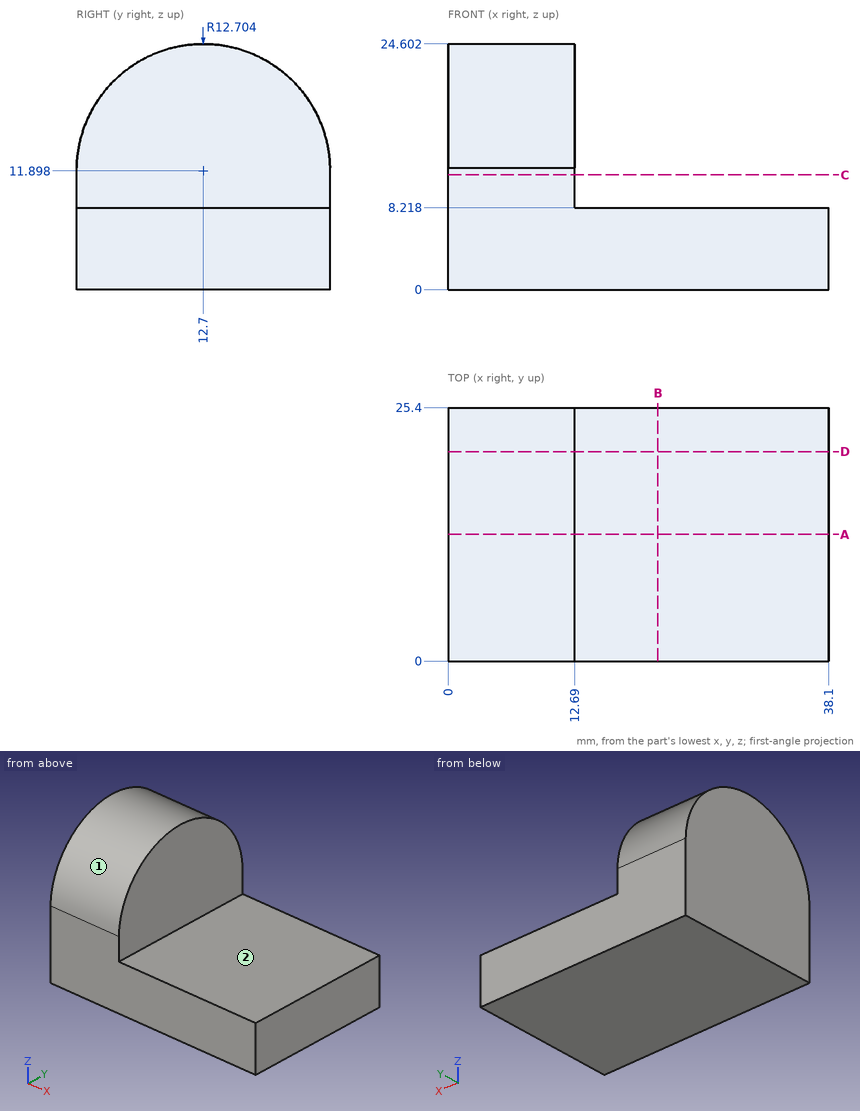
Answer from the drawing. Dimensions are ordinates in mm from the lowest x, y and z of the part. A direction names the side the tool comes from. Give positions to 0.01 mm unless a question says otherwise; leave off trailing zeros. Loops run counter-clockwise (first coordinate to the right, second up) from the corner with the lowest first, then second, coordinate; pieces in that order, holes last. Notation, with made-up numbers: (66, 68.5) -> (72, 68.5) arc R10 cw to (72, 86.5) -> close; hole circle Ø1 at (-24, -33.75). An arc over 180 degrees is marked (long way). One line per question, with ' | ' between items. Start each with the question number.
1) Section C-C, the plane z = 11.5 is taken. Determine the outline of the cut face in (x, y).
2) Each of these flat-tipped pins is pushed along its axis until it touches: pin 1 (3 mm diameter, centred on y = 21.5, z = 11.5, fed in from +X); pin 2 (2 mm diameter, centred on x = 7.5, y = 10, fed in from +Z); pin 3 (1.5 mm diameter, centred on x = 11, y = 18, fed in from +Z). Where does it stop, or does it pass through?
3) Straight lines are drawn through the part: L1, parallel to X at y = 17.5, z = 19.75; L2, parallel to Z at x = 15.5, y = 12.5; L3, parallel to Y at x = 6, z = 21.75. For each, find the intervals that lie inside material, in ascending order.
4) Section D-D, the plane y = 21 is taken. Determine the outline of the cut face in (x, z) (1 decimal), then the cut area to 3 significant figures.
5) For the marked faces 1 and 2, determine the directions among +Z, -Z, +X, -X, +Y, -Y from which every point of the face is accessible in a straight line to the end or side of a thin tool.
6) Section A-A, the plane y = 12.7 is taken. Determine the outline of the cut face in (x, z), then the cut area to 3 significant figures.
7) Section B-B, the plane x = 21 is taken. Determine the outline of the cut face in (y, z), then the cut area to 3 significant figures.
Resolved:
1) outline: (0, 0) -> (12.69, 0) -> (12.69, 25.4) -> (0, 25.4) -> close
2) pin 1: x = 12.69 | pin 2: z = 24.49 | pin 3: z = 23.76
3) L1: 0 to 12.69 | L2: 0 to 8.22 | L3: 4.68 to 20.72
4) outline: (0, 0) -> (38.1, 0) -> (38.1, 8.2) -> (12.7, 8.2) -> (12.7, 21.5) -> (0, 21.5) -> close | area: 482 mm2
5) face 1: +Z, +X, -X | face 2: +Z, +X, +Y, -Y
6) outline: (0, 0) -> (38.1, 0) -> (38.1, 8.22) -> (12.69, 8.22) -> (12.69, 24.6) -> (0, 24.6) -> close | area: 521 mm2
7) outline: (0, 0) -> (25.4, 0) -> (25.4, 8.22) -> (0, 8.22) -> close | area: 209 mm2
